Model file for the job. Use its own axes, mm. A direction names the side the tool comes from. Round coordinates to 2 decimals unless told otherwise and drop trailing zeros. Write each loop counter-clockwise with the first axis right and the second up, starting at its lowest first coordinate (ties: lowest second). Pieces come first, ordered by that corner, then holes. Notation, with made-up numbers: (48, -16.75) - (98, -16.75) arc R33 cw to (98, 19.25) - close; hole circle Ø7 at (69, -7.5). An arc over 180 degrees is marked (long way). One line per item, written item: value.
from build123d import *

# Parameters (mm, degrees)
BOSS_EXTRUDE1_DEPTH = 5.08
SKETCH2_W           = 5.08
SKETCH2_H           = 15.875
SKETCH2_W_2         = 12.7
SKETCH2_H_2         = 5.08
BOSS_EXTRUDE2_DEPTH = 5.08


with BuildPart() as part:
    # Sketch1 → Boss-Extrude1 (new body)
    with BuildSketch(Plane.XY):
        Polygon((-203.2, 0), (-203.2, 31.75), (-25.4, 73.025), (0, 73.025), (0, 0), align=None)
    boss_extrude1 = extrude(amount=BOSS_EXTRUDE1_DEPTH)

    # Mirror1: Boss-Extrude1 across plane
    add(boss_extrude1.mirror(Plane(origin=(0, 73.025, 5.08), x_dir=(0, 0, 1), z_dir=(-1, 0, 0))))

    # Sketch2 → Boss-Extrude2 (add)
    with BuildSketch(Plane.XY.offset(5.08)):
        Polygon((-126.671034443, 49.515652719), (-101.928965557, 55.259347281), (-103.077704469, 60.207761059), (-127.819773356, 54.464066496), align=None)
        with Locations((-205.74, 7.9375)):
            Rectangle(SKETCH2_W, SKETCH2_H)
        with Locations((0, 75.565)):
            Rectangle(SKETCH2_W_2, SKETCH2_H_2)
        with Locations((205.74, 7.9375)):
            Rectangle(SKETCH2_W, SKETCH2_H)
        Polygon((126.671034443, 49.515652719), (101.928965557, 55.259347281), (103.077704469, 60.207761059), (127.819773356, 54.464066496), align=None)
    extrude(amount=-BOSS_EXTRUDE2_DEPTH)


solid = part.part
1. Band-saw the part on B-B on x = -19. Write the cut outline in (y, z) (3 decimals).
Report:
outline: (0, 0) - (73.025, 0) - (73.025, 5.08) - (0, 5.08) - close
2. Band-saw the part on C-C on y = 23. Write the cut outline in (x, z).
Report:
outline: (-203.2, 0) - (203.2, 0) - (203.2, 5.08) - (-203.2, 5.08) - close
3. Wall check: probe 1 along X at (y, z) = (18.5, 3.35); probe 2 along Y at (x, z) = (20.5, 3.6) (3 decimals); probe 3 along X at (y, z) = (73.5, 2.55). Give the ranges that are in metal, low to high. Write a range as [from, to].
Report:
probe 1: [-203.2, 203.2]
probe 2: [0, 73.025]
probe 3: [-6.35, 6.35]
4. Mould opens along X. For faces 3 (the face through (-3, 31, 0)), 4 (the face through (64.2, 64.018, 2.504)), 5 (the face through (-165.5, 40.5, 2.5)) say: released by +X, released by -X, zero draft, split by the parting line, or undercut.
Report:
face 3: zero draft
face 4: undercut
face 5: released by -X
5. Drop flat-ended pins along their axis: pin 1 (1.5 mm diameter, centred on x = 135.5, z = 1.5, fed in from +Y); pin 2 (1.5 mm diameter, centred on y = 74.5, z = 1.5, fed in from -X); pin 3 (1.5 mm diameter, centred on y = 76, z = 1.5, fed in from +X). Give the stop position or say it passes through.
Report:
pin 1: y = 47.64
pin 2: x = -6.35
pin 3: x = 6.35
6. Band-saw the part on A-A on z = 4.3. Write the cut outline in (x, y) (3 decimals), plus the area to 3 significant figures.
Report:
outline: (-208.28, 0) - (208.28, 0) - (208.28, 15.875) - (203.2, 15.875) - (203.2, 31.75) - (126.671, 49.516) - (127.82, 54.464) - (103.078, 60.208) - (101.929, 55.259) - (25.4, 73.025) - (6.35, 73.025) - (6.35, 78.105) - (-6.35, 78.105) - (-6.35, 73.025) - (-25.4, 73.025) - (-101.929, 55.259) - (-103.078, 60.208) - (-127.82, 54.464) - (-126.671, 49.516) - (-203.2, 31.75) - (-203.2, 15.875) - (-208.28, 15.875) - close
area: 22,800 mm²
7. Tool access for faces 1 (the face through (-3, 31, 5.08)), 2 (the face through (-64.2, 64.018, 2.504)): list every direction of +Z, -Z, +X, -X, +Y, -Y with a clear straight run to the whole face (end or side of a thin tool).
Report:
face 1: +Z, +X, -X, +Y, -Y
face 2: +Z, -Z, +Y
